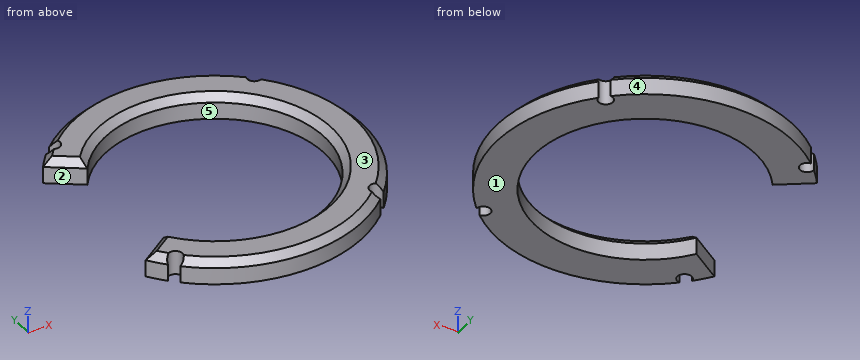
Autodesk Inventor part; units mm, degrees
ref_plane "YZ Plane" through (0, 0, 0) normal (1, 0, 0) x (0, 1, 0)
ref_plane "XZ Plane" through (0, 0, 0) normal (0, 1, 0) x (-1, 0, 0)
ref_plane "XY Plane" through (0, 0, 0) normal (0, 0, 1) x (1, 0, 0)
sketch "スケッチ1" plane through (0, 0, 0) normal (0, 0, 1) x (1, 0, 0)
  arc A0 (-18.8405, -13.1923) -> (-18.8405, 13.1923) centre (0, 0) ccw
  line L0 (-36.6725, 0) -> (42.2787, 0)
  arc A1 (-25.3937, -17.7809) -> (-25.3937, 17.7809) centre (0, 0) ccw
  line L1 (-25.3937, -17.7809) -> (-18.8405, -13.1923)
  line L2 (-18.8405, 13.1923) -> (-25.3937, 17.7809)
  point P0 (23, 0)
  dimension "d0" = 23
  dimension "d1" = 8
  dimension "d2" = 290
extrude "押し出し1" add sketch "スケッチ1" along normal blind 5
chamfer "面取り1" distance 1.5 angle 45 5 edges at (31, 0, 5) (6.9162, -21.9355, 5) (6.9162, 21.9355, 5) (-22.1171, 15.4866, 5) (-22.1171, -15.4866, 5)
sketch "スケッチ2" plane through (0, 0, 5) normal (0, 0, 1) x (1, 0, 0)
  circle A0 centre (-21.2132, 21.2132) radius 1.5
  circle A1 centre (21.2132, 21.2132) radius 1.5
  circle A2 centre (21.2132, -21.2132) radius 1.5
  circle A3 centre (-21.2132, -21.2132) radius 1.5
  point P0 (0, 0)
extrude "押し出し2" cut sketch "スケッチ2" against normal through all
properties part number "cover"
For this review, take the finished solid that the model builds, in its own axes (mm). Face numbers are marked on the shaded views. A direction names the side the tool comes from. Coordinates: 2 decimals unless noted, no trailing zeros. Order: outer loops, then holes, each group sorted by start corner. A loop starts at its lowest first (then second) coordinate and runs counter-clockwise, first axis right, second up. Notation, with made-up numbers: (-27.5, -12.75) - (11.5, -12.75) arc R36 ccw to (11.5, 24.25) - close; hole circle Ø10 at (-7, 0). An arc over 180 degrees is marked (long way). Answer as CSV lines item,"result". Start each with the question number.
1) Machinability: for the marked faces 1 and 2, which of the approach directions +Z, -Z, +X, -X, +Y, -Y give a long, thin tool a straight path to every point of the face, cutting with its end or side? Answer none if there is none.
2) Draft analysis for pull direction Y (two halves, no side actions). For the marked faces 3, 4 and 5, state which applies: +Y half, -Y half, draft (parallel to the pull), parting line (faces both ways), or undercut.
3) Add section A-A (x = 0). State the section outline as (y, z) points.
4) Add section B-B (y = 0). State the section outline as (x, z) points.
5) Insertion check: P1, Ø2, axis at y = 24, z = 1.5, coming from the +X side; P2, Ø1, axis at y = 14.5, z = 2.5, coming from the -X side; P3, Ø1.5, axis at y = -12, z = 1, coming from the -X side. Each pin has a flat end and moves straight along its axis. Give the tip position at first contact, or say it passes through.
6) To check wall thickness, follow line 1 along Y through (x, z) = (0, 2.4); line 2 along Y through (x, z) = (20, 0.8). State the ranges of each line that lie inside material, in increasing order. Write a range as [from, to].
Result:
1,face 1,"-Z, +X, -X, +Y, -Y"
1,face 2,"+Z, -Z, -X"
2,face 3,"draft"
2,face 4,"+Y half"
2,face 5,"undercut"
3,outline,"(-31, 0) - (-23, 0) - (-23, 3.5) - (-24.5, 5) - (-29.5, 5) - (-31, 3.5) - close; (23, 0) - (31, 0) - (31, 3.5) - (29.5, 5) - (24.5, 5) - (23, 3.5) - close"
4,outline,"(23, 0) - (31, 0) - (31, 3.5) - (29.5, 5) - (24.5, 5) - (23, 3.5) - close"
5,P1,"x = 20.78"
5,P2,"x = -21.42"
5,P3,"x = 19.14"
6,line 1,"[-31, -23], [23, 31]"
6,line 2,"[-23.69, -22.1], [-20.33, -11.36], [11.36, 20.33], [22.1, 23.69]"
